Input: part model. Units: mm. Frame: model coordinates. Coordinates: 2 decimals unless noted, no trailing zeros. Order: outer loops, then holes, each group sorted by start corner. A loop starts at its lowest first (then second) coordinate and runs counter-clockwise, first axis right, second up. Notation, with made-up numbers: (70.5, -7) - (82.5, -7) arc R20 cw to (82.5, 15) - close; hole circle Ø9 at (33, 43). An arc over 180 degrees is marked (long way). Use a Markdown table: item, result. Add a question column.
from build123d import *

# Parameters (mm, degrees)
SKETCH1_W           = 111
SKETCH1_H           = 126.5
BOSS_EXTRUDE1_DEPTH = 6
SKETCH2_W           = 60
SKETCH2_H           = 40
CUT_EXTRUDE1_DEPTH  = 7
FILLET1_R           = 5


with BuildPart() as part:
    # Sketch1 → Boss-Extrude1 (new body)
    with BuildSketch(Plane(origin=(0, 0, 0), x_dir=(1, 0, 0), z_dir=(0, 1, 0))):
        with Locations((55.5, 63.25)):
            Rectangle(SKETCH1_W, SKETCH1_H)
    extrude(amount=BOSS_EXTRUDE1_DEPTH)

    # Sketch2 → Cut-Extrude1 (cut, through all)
    with BuildSketch(Plane(origin=(0, 6, 0), x_dir=(1, 0, 0), z_dir=(0, 1, 0))):
        with Locations((30, 63.25)):
            Rectangle(SKETCH2_W, SKETCH2_H)
    extrude(amount=-CUT_EXTRUDE1_DEPTH, mode=Mode.SUBTRACT)

    # Fillet1
    fillet1_edges = [part.edges().sort_by_distance(p)[0] for p in [
        (60, 3, -83.25),
        (60, 3, -43.25),
    ]]
    fillet(fillet1_edges, radius=FILLET1_R)


solid = part.part
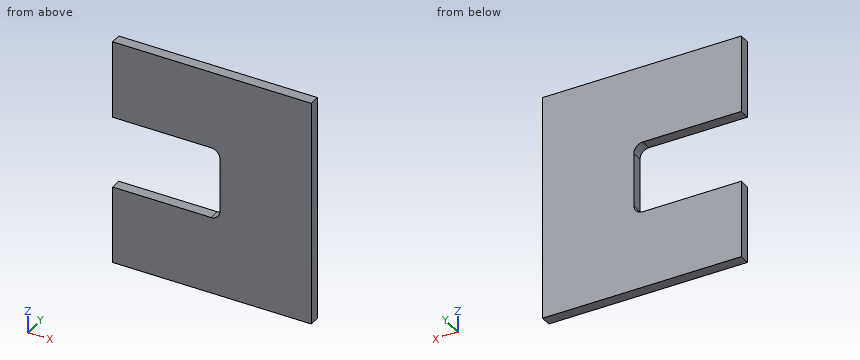
1) Contact query for a flat-ended pin moving along its axis: P1, Ø3, axis at y = 1.5, z = -58, coming from the -X side. Output: stop coordinate, or through.
2) Cut plane B-B (y = 2.35). Return the cut outline in (x, z).
3) Cut plane C-C (z = -72). Return the cut outline in (x, y).
4) Material intervals for L1, parallel to Z at x = 17, y = 4.75; L2, parallel to X at y = 3.95, z = -72; L3, parallel to Z at x = 57.5, y = 0.4, sorted ascending.
5) Cut plane A-A (x = 45.5). Return the cut outline in (y, z), and give its area (3 significant figures).
Computed:
| question | item | result |
|---|---|---|
| 1 | P1 | stops at x = 60 |
| 2 | outline | (0, -126.5) - (111, -126.5) - (111, 0) - (0, 0) - (0, -43.25) - (55, -43.25) arc R5 cw to (60, -48.25) - (60, -78.25) arc R5 cw to (55, -83.25) - (0, -83.25) - close |
| 3 | outline | (60, 0) - (111, 0) - (111, 6) - (60, 6) - close |
| 4 | L1 | z = -126.5 to -83.25, -43.25 to 0 |
| 4 | L2 | x = 60 to 111 |
| 4 | L3 | z = -126.5 to -82.58, -43.92 to 0 |
| 5 | outline | (0, -126.5) - (6, -126.5) - (6, -83.25) - (0, -83.25) - close; (0, -43.25) - (6, -43.25) - (6, 0) - (0, 0) - close |
| 5 | area | 519 mm2 |
